Geometry: final body of the model. Coordinates: model frame, mm. A direction names the side the tool comes from. Round coordinates to 2 decimals unless told otherwise and drop trailing zeros. Loops run counter-clockwise (first coordinate to the right, second up) from the corner with the lowest first, then second, coordinate; pieces in that order, holes last. Notation, with made-up numbers: (80.25, 61.25) - (136.25, 61.25) arc R30 ccw to (136.25, 91.25) - close; hole circle Ø10 at (-8.5, -18). An arc over 180 degrees is marked (long way). Return JSON: item names as keys, results as strings. Group by question number.
1. Section A-A on z = 25. Return loops of the section in (x, y), and give its area (3 significant figures).
2. Section D-D on y = -70. Count the separate pieces of the cut face and the enclosed holes in it, and give its area (3 significant figures).
3. Section B-B on y = -7.5. Return loops of the section in (x, z), and give its area (3 significant figures).
4. First-contact query: pin 1 Ø5 at (x, y) = (20, -7.5) entering from +Z; pin 2 Ø4 at (y, z) = (-70, 40) entering from +X; pin 3 Ø12 at (x, y) = (18.5, -42) entering from +Z; pin 4 Ø3.5 at (x, y) = (20, -37.5) entering from -Z. Flat tips, straight axial feed; report the tip coordinate or a pass-through.
5. Section C-C on x = 0. Return loops of the section in (y, z), and give its area (3 significant figures).
6. Draft query along Y for faces 1 (the face through (35.56, -70.46, 37.95)), 2 (the face through (31, -72.3, 38.8)), 3 (the face through (-22.21, -5.47, 12.01)), 4 (the face through (1, -15, 3)). Return one class per face: +Y half, -Y half, draft (parallel to the pull), parting line (faces both ways), or undercut.
7. Material intervals for probe 1 along X at (y, z) = (-68.65, 25); probe 2 along Z at (x, y) = (26.4, -70); probe 3 along X at (y, z) = (-65.5, 22.5), sorted ascending.
8. Set-up query: faces 5 (the face through (3.38, -68.04, 14.27)), 6 (the face through (-26.284, -68.722, 41.666)), 7 (the face through (-14, -70, 46)). Return all of +Z, -Z, +X, -X, +Y, -Y with unobstructed straight access to the full face (end or side cutting, diameter ignored); none if empty.
from build123d import *

# Parameters (mm, degrees)
SKETCH_1_W           = 80
SKETCH_1_H           = 150
EXTRUDE_1_DEPTH      = 10
SKETCH_4_R           = 11.25
EXTRUDE_3_DEPTH      = 10
SKETCH_5_R           = 11.25
SKETCH_5_R_2         = 5
EXTRUDE_4_DEPTH      = 4
SKETCH_6_R           = 2.1
CUT_EXTRUDE_1_DEPTH  = 24
SKETCH_7_W           = 3.4
SKETCH_7_H           = 7.5
CUT_EXTRUDE_2_DEPTH  = 24
CUT_EXTRUDE_START    = -24
SKETCH_8_R           = 2.1
CUT_EXTRUDE_3_DEPTH  = 24
SKETCH_9_W           = 80
SKETCH_9_H           = 40
SKETCH_9_R           = 11
SKETCH_9_R_2         = 1.6
EXTRUDE_5_DEPTH      = 10
FILLET_1_R           = 5
CUT_EXTRUDE_START_2  = -10
SKETCH_10_W          = 3.4
SKETCH_10_H          = 7.5
CUT_EXTRUDE_5_DEPTH  = 10
SKETCH_11_R          = 2.1
CUT_EXTRUDE_6_DEPTH  = 24
SKETCH_12_R          = 2.1
CUT_EXTRUDE_7_DEPTH  = 24
SKETCH_14_W          = 4
SKETCH_14_H          = 2
CUT_EXTRUDE_9_DEPTH  = 10
SKETCH_16_R          = 2.1
CUT_EXTRUDE_10_DEPTH = 94.94147114
CUT_EXTRUDE_11_DEPTH = 121.519707932
SKETCH_18_W          = 3
SKETCH_18_H          = 15
EXTRUDE_7_DEPTH      = 80
FILLET_2_R           = 10
SKETCH_19_R          = 1.6
CUT_EXTRUDE_12_DEPTH = 80
SKETCH_20_R          = 3
CUT_EXTRUDE_13_DEPTH = 2


with BuildPart() as part:
    # 草圖1 → 填料-伸長1 (new body)
    with BuildSketch(Plane.XY):
        Rectangle(SKETCH_1_W, SKETCH_1_H)
    extrude(amount=EXTRUDE_1_DEPTH)

    # 草圖4 → 填料-伸長3 (add)
    with BuildSketch(Plane.XZ.offset(75)):
        with BuildLine():
            ThreePointArc((-6, 49), (0, 43), (6, 49))
            Line((6, 49), (6, 50))
            Line((6, 50), (29, 50))
            Line((29, 50), (29, 27.881405907))
            ThreePointArc((29, 27.881405907), (30, 21.95), (31, 27.881405907))
            Line((31, 27.881405907), (31, 50))
            Line((31, 50), (40, 50))
            Line((40, 50), (40, 10))
            Line((40, 10), (-40, 10))
            Line((-40, 10), (-40, 50))
            Line((-40, 50), (-31, 50))
            Line((-31, 50), (-31, 27.881405907))
            ThreePointArc((-31, 27.881405907), (-30, 21.95), (-29, 27.881405907))
            Line((-29, 27.881405907), (-29, 50))
            Line((-29, 50), (-6, 50))
            Line((-6, 50), (-6, 49))
        make_face()
        with Locations(Location((0, 25, 0), (0, 0, 270))):
            Circle(SKETCH_4_R, mode=Mode.SUBTRACT)
    extrude(amount=-EXTRUDE_3_DEPTH)

    # 草圖5 → 填料-伸長4 (add)
    with BuildSketch(Plane.XZ.offset(75)):
        with Locations(Location((0, 25, 0), (0, 0, 270))):
            Circle(SKETCH_5_R)
        with Locations(Location((0, 25, 0), (0, 0, 270))):
            Circle(SKETCH_5_R_2, mode=Mode.SUBTRACT)
    extrude(amount=-EXTRUDE_4_DEPTH)

    # 草圖6 → 除料-伸長1 (cut)
    with BuildSketch(Plane(origin=(40, 0, 0), x_dir=(0, 0, -1), z_dir=(1, 0, 0))):
        with Locations(Location((-40, -70, 0), (0, 0, 90))):
            Circle(SKETCH_6_R)
    extrude(amount=-CUT_EXTRUDE_1_DEPTH, mode=Mode.SUBTRACT)

    # 草圖7 → 除料-伸長2 (cut)
    with BuildSketch(Plane.XZ.offset(75)):
        with Locations((-21.943112787, 40)):
            Rectangle(SKETCH_7_W, SKETCH_7_H)
        with Locations((21.943112787, 40)):
            Rectangle(SKETCH_7_W, SKETCH_7_H)
    extrude(amount=-CUT_EXTRUDE_2_DEPTH, mode=Mode.SUBTRACT)

    # 草圖8 → 除料-伸長3 (cut)
    with BuildSketch(Plane.ZY.offset(40).offset(CUT_EXTRUDE_START)):
        with Locations(Location((40, -70, 0), (0, 0, 180))):
            Circle(SKETCH_8_R)
    extrude(amount=CUT_EXTRUDE_3_DEPTH, mode=Mode.SUBTRACT)

    # 草圖9 → 填料-伸長5 (add)
    with BuildSketch(Plane(origin=(0, 75, 0), x_dir=(1, 0, 0), z_dir=(0, 1, 0))):
        with Locations((0, -30)):
            Rectangle(SKETCH_9_W, SKETCH_9_H)
        with Locations(Location((0, -25, 0), (0, 0, 270))):
            Circle(SKETCH_9_R, mode=Mode.SUBTRACT)
        with Locations(Location((-21.920310217, -25, 0), (0, 0, 270))):
            Circle(SKETCH_9_R_2, mode=Mode.SUBTRACT)
        with Locations(Location((0, -46.920310217, 0), (0, 0, 270))):
            Circle(SKETCH_9_R_2, mode=Mode.SUBTRACT)
        with Locations(Location((21.920310217, -25, 0), (0, 0, 270))):
            Circle(SKETCH_9_R_2, mode=Mode.SUBTRACT)
    extrude(amount=-EXTRUDE_5_DEPTH)

    # 圓角1
    fillet_1_edges = [part.edges().sort_by_distance(p)[0] for p in [
        (40, 70, 50),
        (-40, 70, 50),
        (40, -70, 50),
        (-40, -70, 50),
    ]]
    fillet(fillet_1_edges, radius=FILLET_1_R)

    # 草圖10 → 除料-伸長5 (cut)
    with BuildSketch(Plane(origin=(0, 75, 0), x_dir=(1, 0, 0), z_dir=(0, 1, 0)).offset(CUT_EXTRUDE_START_2)):
        with BuildLine():
            Line((-30.992105359, -72.117230176), (-29, -72.117230176))
            Line((-29, -72.117230176), (-29, -27.881405907))
            ThreePointArc((-29, -27.881405907), (-30.004176302, -21.950002859), (-30.992105359, -27.884133658))
            Line((-30.992105359, -27.884133658), (-30.992105359, -72.117230176))
        make_face()
        with BuildLine():
            Line((29.001577897, -72.118320527), (31, -72.118320527))
            Line((31, -72.118320527), (31, -27.881405907))
            ThreePointArc((31, -27.881405907), (29.999164969, -21.950000114), (29.001577897, -27.881953036))
            Line((29.001577897, -27.881953036), (29.001577897, -72.118320527))
        make_face()
        with Locations((-21.943112787, -40)):
            Rectangle(SKETCH_10_W, SKETCH_10_H)
        with Locations((21.943112787, -40)):
            Rectangle(SKETCH_10_W, SKETCH_10_H)
    extrude(amount=CUT_EXTRUDE_5_DEPTH, mode=Mode.SUBTRACT)

    # 草圖11 → 除料-伸長6 (cut)
    with BuildSketch(Plane(origin=(40, 0, 0), x_dir=(0, 0, -1), z_dir=(1, 0, 0))):
        with Locations((-40, 70)):
            Circle(SKETCH_11_R)
    extrude(amount=-CUT_EXTRUDE_6_DEPTH, mode=Mode.SUBTRACT)

    # 草圖12 → 除料-伸長7 (cut)
    with BuildSketch(Plane.ZY.offset(40).offset(CUT_EXTRUDE_START)):
        with Locations(Location((40, 70, 0), (0, 0, 180))):
            Circle(SKETCH_12_R)
    extrude(amount=CUT_EXTRUDE_7_DEPTH, mode=Mode.SUBTRACT)

    # 草圖14 → 除料-伸長9 (cut)
    with BuildSketch(Plane.XZ.offset(75)):
        with Locations((-12, 46)):
            Rectangle(SKETCH_14_W, SKETCH_14_H)
        with Locations((12, 46)):
            Rectangle(SKETCH_14_W, SKETCH_14_H)
    extrude(amount=-CUT_EXTRUDE_9_DEPTH, mode=Mode.SUBTRACT)

    # 草圖16 → 除料-伸長10 (cut, through all)
    with BuildSketch(Plane.XY.offset(10)):
        with Locations((-20, 37.5)):
            Circle(SKETCH_16_R)
        with Locations((20, 37.5)):
            Circle(SKETCH_16_R)
        with Locations((20, -37.5)):
            Circle(SKETCH_16_R)
        with Locations((-20, -37.5)):
            Circle(SKETCH_16_R)
    extrude(amount=-CUT_EXTRUDE_10_DEPTH, mode=Mode.SUBTRACT)

    # 草圖17 → 除料-伸長11 (cut, through all)
    with BuildSketch(Plane(origin=(40, 0, 0), x_dir=(0, 0, -1), z_dir=(1, 0, 0))):
        Polygon((-5, 0), (-5, -15), (0, -15), (0, 75), (-50, 75), (-50, 65), (-10, 65), (-10, 0), align=None)
    extrude(amount=-CUT_EXTRUDE_11_DEPTH, mode=Mode.SUBTRACT)

    # 草圖18 → 填料-伸長7 (add)
    with BuildSketch(Plane(origin=(40, 0, 0), x_dir=(0, 0, -1), z_dir=(1, 0, 0))):
        with Locations((-11.5, -7.5)):
            Rectangle(SKETCH_18_W, SKETCH_18_H)
    extrude(amount=-EXTRUDE_7_DEPTH)

    # 圓角2
    # the kernel refuses this fillet: 10 mm, written as the material it adds along each edge
    with BuildSketch(Plane(origin=(40, -15, 10), x_dir=(0, 0, 1), z_dir=(-1, 0, 0))) as fillet_2_piece_1:
        with BuildLine():
            CenterArc((10, -7.141428429), FILLET_2_R, 134.427004001, 45.572995999)
            Line((0, -7.141428429), (-0.2, -7.141428429))
            Line((-0.2, -7.141428429), (-0.2, 0))
            Line((-0.2, 0), (0, 0.2))
            ThreePointArc((0, 0.2), (1.5, 0.2), (2.86, 0.142828569))
            Line((2.86, 0.142828569), (3, 0))
        make_face()
    extrude(amount=80)

    # 草圖19 → 除料-伸長12 (cut)
    with BuildSketch(Plane.XY.offset(13)):
        with Locations((-20, -7.5)):
            Circle(SKETCH_19_R)
        with Locations(Location((20, -7.5, 0), (0, 0, 270))):
            Circle(SKETCH_19_R)
    extrude(amount=-CUT_EXTRUDE_12_DEPTH, mode=Mode.SUBTRACT)

    # 草圖20 → 除料-伸長13 (cut)
    with BuildSketch(Plane.XY.offset(13)):
        with Locations((-20, -7.5)):
            Circle(SKETCH_20_R)
        with Locations((20, -7.5)):
            Circle(SKETCH_20_R)
    extrude(amount=-CUT_EXTRUDE_13_DEPTH, mode=Mode.SUBTRACT)


solid = part.part
Taken from the geometry:
{
 "1": {"outline": "(-40, -75) - (-33.05, -75) - (-33.05, -65) - (-40, -65) - close; (-26.95, -75) - (-5, -75) - (-5, -71) - (-11.25, -71) - (-11.25, -65) - (-26.95, -65) - close; (5, -75) - (26.95, -75) - (26.95, -65) - (11.25, -65) - (11.25, -71) - (5, -71) - close; (33.05, -75) - (40, -75) - (40, -65) - (33.05, -65) - close", "area": "503 mm2"},
 "2": {"separate pieces": "3", "enclosed holes": "3", "area": "3,150 mm2"},
 "3": {"outline": "(-40, 5) - (-21.6, 5) - (-21.6, 11) - (-23, 11) - (-23, 13) - (-40, 13) - close; (-18.4, 5) - (18.4, 5) - (18.4, 11) - (17, 11) - (17, 13) - (-17, 13) - (-17, 11) - (-18.4, 11) - close; (21.6, 5) - (40, 5) - (40, 13) - (23, 13) - (23, 11) - (21.6, 11) - close", "area": "578 mm2"},
 "4": {"pin 1": "z = 11", "pin 2": "x = 16", "pin 3": "z = 10", "pin 4": "through"},
 "5": {"outline": "(-75, 0) - (-15, 0) - (-15, 5) - (0, 5) - (0, 13) - (-15, 13) arc R10 cw to (-22.14, 10) - (-65, 10) - (-65, 13.75) - (-71, 13.75) - (-71, 20) - (-75, 20) - close; (-75, 30) - (-71, 30) - (-71, 36.25) - (-65, 36.25) - (-65, 43) - (-75, 43) - close", "area": "882 mm2"},
 "6": {"face 1": "undercut", "face 2": "draft", "face 3": "undercut", "face 4": "+Y half"},
 "7": {"probe 1": "-40 to -33.05, -26.95 to -11.25, 11.25 to 26.95, 33.05 to 40", "probe 2": "0 to 37.9, 42.1 to 50", "probe 3": "-40 to -31.75, -28.25 to -10.97, 10.97 to 28.25, 31.75 to 40"},
 "8": {"face 5": "+Y", "face 6": "-X", "face 7": "+Y, -Y"}
}
